Check sheet for the modelled part. Datum: model origin and axes. Units: mm. A direction names the side the tool comes from. Give positions to 0.01 mm unless a question says otherwise; leave off trailing zeros. Order: outer loops, then holes, each group sorted by start corner. A loop starts at its lowest first (then second) coordinate and runs counter-clockwise, first axis right, second up.
Item 1: Gauge pin test, flat ends, axial feed: P1, Ø0.6, axis at y = 0.5, z = -14.5, coming from the +X side; P2, Ø1, axis at x = 3.5, y = 1, coming from the -Z side; P3, Ø2.5, axis at x = 4.15, z = -3, coming from the -Y side. Record the tip position at first contact, or that the pin passes through.
Item 2: Sectioned sample at D-D on y = 0.85. Record the boundary of the cut face in (x, z), and give its area (3 significant figures).
Item 3: Sectioned sample at C-C on x = 31.5. Record the boundary of the cut face in (y, z).
Item 4: Material ranges on line 1 along X through (y, z) = (1.25, -26.5); line 2 along Z through (x, y) = (30, 0.4); line 3 along X through (y, z) = (0.35, -20), recorded low to high.
Item 5: Sectioned sample at A-A on x = 4.15. Record the boundary of the cut face in (y, z), and give its area (3 significant figures).
Item 6: Release check for a two-part mould opening along Z. For faces 4 (the flat face through (17, 1, 0)), 5 (the cylindrical face through (34.638, 1.014, -11.618)), 6 (the flat face through (35, 1, -6)) record: released by +Z, released by -Z, zero draft, split by the parting line, or undercut.
Item 7: Access from +Z, -Z, +X, -X, +Y, -Y to the whole of each face (thin tool, end or side, straight path). Record for faces 1 (the cylindrical face through (34.618, 1.014, -0.362)), 2 (the flat face through (8, 1, -19)), 3 (the flat face through (30, 1, -12)).
Item 8: Sectioned sample at B-B on z = -3. Record the boundary of the cut face in (x, y).
from build123d import *

# Parameters (mm, degrees)
CROQUIS1_R              = 2
SALIENTE_EXTRUIR1_DEPTH = 2
REDONDEO5_R             = 1.27


with BuildPart() as part:
    # Croquis1 → Saliente-Extruir1 (new body)
    with BuildSketch(Plane(origin=(0, 0, 0), x_dir=(1, 0, 0), z_dir=(0, 1, 0))):
        Polygon((0, 0), (35, 0), (35, 12), (25, 12), (25, 17.5), (35, 17.5), (35, 29.5), (8, 29.5), (8, 7.5), (0, 7.5), align=None)
        with Locations(Location((4.15, 3, 0), (0, 0, 270))):
            Circle(CROQUIS1_R, mode=Mode.SUBTRACT)
        with Locations(Location((31.5, 26.5, 0), (0, 0, 270))):
            Circle(CROQUIS1_R, mode=Mode.SUBTRACT)
    extrude(amount=SALIENTE_EXTRUIR1_DEPTH)

    # Redondeo5
    redondeo5_edges = [part.edges().sort_by_distance(p)[0] for p in [
        (0, 1, -7.5),
        (8, 1, -7.5),
        (8, 1, -29.5),
        (35, 1, -29.5),
        (35, 1, -17.5),
        (25, 1, -17.5),
        (25, 1, -12),
        (35, 1, -12),
        (35, 1, 0),
        (0, 1, 0),
    ]]
    fillet(redondeo5_edges, radius=REDONDEO5_R)


solid = part.part
Report:
1. P1: stops at x = 25
1. P2: stops at z = -7.5
1. P3: passes through
2. outline: (0, -6.23) arc R1.27 ccw to (1.27, -7.5) - (6.73, -7.5) arc R1.27 cw to (8, -8.77) - (8, -28.23) arc R1.27 ccw to (9.27, -29.5) - (33.73, -29.5) arc R1.27 ccw to (35, -28.23) - (35, -18.77) arc R1.27 ccw to (33.73, -17.5) - (26.27, -17.5) arc R1.27 cw to (25, -16.23) - (25, -13.27) arc R1.27 cw to (26.27, -12) - (33.73, -12) arc R1.27 ccw to (35, -10.73) - (35, -1.27) arc R1.27 ccw to (33.73, 0) - (1.27, 0) arc R1.27 ccw to (0, -1.27) - close; hole circle Ø4 at (4.15, -3); hole circle Ø4 at (31.5, -26.5)
2. area: 775 mm2
3. outline: (0, -29.5) - (2, -29.5) - (2, -28.5) - (0, -28.5) - close; (0, -24.5) - (2, -24.5) - (2, -17.5) - (0, -17.5) - close; (0, -12) - (2, -12) - (2, 0) - (0, 0) - close
4. line 1: x = 8 to 29.5, 33.5 to 35
4. line 2: z = -29.5 to -27.82, -25.18 to -17.5, -12 to 0
4. line 3: x = 8 to 35
5. outline: (0, -7.5) - (2, -7.5) - (2, -5) - (0, -5) - close; (0, -1) - (2, -1) - (2, 0) - (0, 0) - close
5. area: 7.00 mm2
6. face 4: released by +Z
6. face 5: undercut
6. face 6: zero draft
7. face 1: +Z, +X, +Y, -Y
7. face 2: -Z, -X, +Y, -Y
7. face 3: +X, +Y, -Y
8. outline: (0, 0) - (2.15, 0) - (2.15, 2) - (0, 2) - close; (6.15, 0) - (35, 0) - (35, 2) - (6.15, 2) - close
